Read the model definition and answer for the solid it produces. Units are mm, in the model's axes. Coordinates: 2 decimals unless noted, no trailing zeros. Order: outer loops, then holes, each group sorted by start corner. A loop starts at its lowest first (then second) coordinate and runs counter-clockwise, first axis right, second up. Notation, with made-up numbers: M -4,5 L 31,5 A21 cw 31,20 Z; hole C -33.75,66 d9. An arc over 180 degrees is marked long. Use a Markdown table: item, result. Add a question column.
1) This flat-tipped pin is pushed along its axis until it touches: pin 1 Ø3 at (x, y) = (36, -23.5) entering from -Z. Where does it stop, or does it pass through?
2) Find section A-A on z = 0.6. Count the separate pieces of the cut face and the enclosed holes in it, plus the area to 3 significant figures.
3) Find section B-B on y = -11.5. Write down the section's boundary in (x, z).
4) Find the intervals of material crossed by probe 1 along Y at (x, z) = (-28, 0.45); probe 2 along Y at (x, z) = (36, 0.8); probe 3 along X at (y, z) = (9, 0.45), in increasing order. Write a range as [from, to].
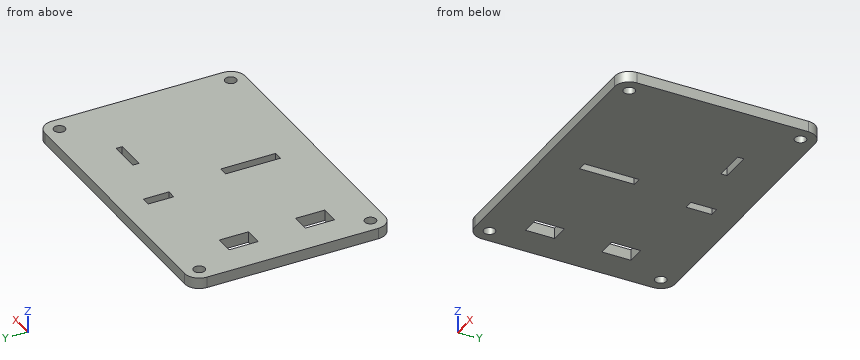
from build123d import *

# Parameters (mm, degrees)
ESQUISSE1_R        = 1.55
ESQUISSE1_W        = 5
ESQUISSE1_H        = 8
ESQUISSE1_W_2      = 2.5
ESQUISSE1_H_2      = 15
ESQUISSE1_H_3      = 7
ESQUISSE1_W_3      = 8.6
ESQUISSE1_H_4      = 1.65
BOSS_EXTRU_1_DEPTH = 3


with BuildPart() as part:
    # Esquisse1 → Boss.-Extru.1 (new body)
    with BuildSketch(Plane.XY):
        with BuildLine():
            Line((36, 27.5), (-36, 27.5))
            ThreePointArc((-36, 27.5), (-38.828427125, 26.328427125), (-40, 23.5))
            Line((-40, 23.5), (-40, -23.5))
            ThreePointArc((-40, -23.5), (-38.828427125, -26.328427125), (-36, -27.5))
            Line((-36, -27.5), (36, -27.5))
            ThreePointArc((36, -27.5), (38.828427125, -26.328427125), (40, -23.5))
            Line((40, -23.5), (40, 23.5))
            ThreePointArc((40, 23.5), (38.828427125, 26.328427125), (36, 27.5))
        make_face()
        with Locations((-36, 23.5)):
            Circle(ESQUISSE1_R, mode=Mode.SUBTRACT)
        with Locations((-36, -23.5)):
            Circle(ESQUISSE1_R, mode=Mode.SUBTRACT)
        with Locations((36, -23.5)):
            Circle(ESQUISSE1_R, mode=Mode.SUBTRACT)
        with Locations((36, 23.5)):
            Circle(ESQUISSE1_R, mode=Mode.SUBTRACT)
        with Locations((-29.1, -12)):
            Rectangle(ESQUISSE1_W, ESQUISSE1_H, mode=Mode.SUBTRACT)
        with Locations((-29.1, 9)):
            Rectangle(ESQUISSE1_W, ESQUISSE1_H, mode=Mode.SUBTRACT)
        with Locations((0.4, -10)):
            Rectangle(ESQUISSE1_W_2, ESQUISSE1_H_2, mode=Mode.SUBTRACT)
        with Locations((-2.85, 17)):
            Rectangle(ESQUISSE1_W_2, ESQUISSE1_H_3, mode=Mode.SUBTRACT)
        with Locations((17.5, 14.675)):
            Rectangle(ESQUISSE1_W_3, ESQUISSE1_H_4, mode=Mode.SUBTRACT)
    extrude(amount=BOSS_EXTRU_1_DEPTH)


solid = part.part
Check result:
| question | item | result |
|---|---|---|
| 1 | pin 1 | passes through |
| 2 | separate pieces | 1 |
| 2 | enclosed holes | 9 |
| 2 | area | 4,210 mm2 |
| 3 | outline | M -40,0 L -31.6,0 L -31.6,3 L -40,3 Z; M -26.6,0 L -0.85,0 L -0.85,3 L -26.6,3 Z; M 1.65,0 L 40,0 L 40,3 L 1.65,3 Z |
| 4 | probe 1 | y = [-27.5, -16], [-8, 5], [13, 27.5] |
| 4 | probe 2 | y = [-27.5, -25.05], [-21.95, 21.95], [25.05, 27.5] |
| 4 | probe 3 | x = [-40, -31.6], [-26.6, 40] |
